Autodesk Inventor part; units mm, degrees
ref_plane "YZ Plane" through (0, 0, 0) normal (1, 0, 0) x (0, 1, 0)
ref_plane "XZ Plane" through (0, 0, 0) normal (0, 1, 0) x (-1, 0, 0)
ref_plane "XY Plane" through (0, 0, 0) normal (0, 0, 1) x (1, 0, 0)
sketch "スケッチ1" plane through (0, 0, 0) normal (0, 1, 0) x (-1, 0, 0)
  line L0 (0, 0) -> (70, 0)
  line L1 (70, 0) -> (70, -170)
  line L2 (70, -170) -> (0, -170)
  line L3 (0, -170) -> (0, 0)
  arc A0 (0, -118.9591) -> (0, -26.9591) centre (0, -72.9591) ccw
  arc A1 (0, -128.9591) -> (0, -16.9591) centre (0, -72.9591) ccw
  line L4 (10, -17.8592) -> (0, -17.8592)
  line L5 (0, -17.8592) -> (0, -2.8592)
  line L6 (0, -2.8592) -> (10, -2.8592)
  line L7 (10, -2.8592) -> (10, -17.8592)
  line L8 (10, -128.0591) -> (0, -128.0591)
  line L9 (0, -128.0591) -> (0, -143.0591)
  line L10 (0, -143.0591) -> (10, -143.0591)
  line L11 (10, -143.0591) -> (10, -128.0591)
  line L12 (54.5871, -60.4591) -> (54.5871, -85.4591)
  point P0 (54.5871, -72.9591)
  point P1 (46, -72.9591)
  dimension "d8" = 70
  dimension "d9" = 170
  dimension "d10" = 46
  dimension "d11" = 56
  dimension "d12" = 10
  dimension "d13" = 10
  dimension "d14" = 15
  dimension "d15" = 15
  dimension "d17" = 25
extrude "押し出し1" add sketch "スケッチ1" along normal blind 81 contours L6 L7 A1 L3 | A1 L4 L3 | L4 A1 L12 L8 L3 A0 | L3 A1 L11 L10 | L3 L8 A1
ref_plane "作業平面1" through (-54.5871, 0, -85.4591) normal (-1, 0, 0) x (0, 0, 1)
sketch "スケッチ2" plane through (-54.5871, 0, -85.4591) normal (-1, 0, 0) x (0, 0, 1)
  line L0 (-33.5, 81) -> (58.5, 81)
  line L1 (0, 60.4) -> (25, 60.4)
  line L2 (25, 60.4) -> (25, 0)
  line L3 (25, 0) -> (0, 0)
  line L4 (0, 0) -> (0, 60.4)
  line L5 (0, 81) -> (25, 81)
  line L6 (0, 0) -> (0, 81)
  line L7 (0, 0) -> (25, 0)
  line L8 (-57.5999, 0) -> (-57.5999, 81)
  line L9 (82.5999, 0) -> (82.5999, 81)
  line L10 (-57.5999, 81) -> (82.5999, 0)
  line L11 (-57.5999, 0) -> (-42.5999, 0)
  line L12 (-57.5999, 0) -> (82.5999, 81)
  line L13 (12.5, 40.5) -> (12.5, 0) construction
  point P0 (85.4591, 0)
  point P1 (12.5, 81)
  point P2 (12.5, 81)
  point P3 (0, 40.5)
  dimension "d21" = 25
  dimension "d22" = 60.4
  dimension "d50" = 20.6
  dimension "d92" = 40.5
  dimension "d93" = 40.5
  dimension "d96" = 12.5
extrude "押し出し2" add sketch "スケッチ2" along normal blind 30 contours L1 L2 L12 L10 L4 | L10 L12 L4 | L2 L10 L12 | L12 L10 L2 L3 L4
ref_plane "作業平面3" through (-84.5871, 0, -85.4591) normal (-1, 0, 0) x (0, 0, 1)
sketch "スケッチ4" plane through (-84.5871, 0, -85.4591) normal (-1, 0, 0) x (0, 0, 1)
  line L0 (2.45, 50.4) -> (22.55, 50.4)
  line L1 (22.55, 50.4) -> (22.55, 10.4)
  line L2 (22.55, 10.4) -> (2.45, 10.4)
  line L3 (2.45, 10.4) -> (2.45, 50.4)
  line L4 (0, 60.4) -> (25, 60.4)
  line L5 (0, 0) -> (0, 60.4)
  line L6 (0, 60.4) -> (0, 0)
  line L7 (0, 0) -> (25, 0)
  line L8 (7.6, 54.5) -> (17.3, 54.5)
  line L9 (7.7, 6.3) -> (17.4, 6.3)
  line L10 (25, 60.4) -> (0, 60.4)
  line L11 (0, 81) -> (25, 81)
  line L12 (25, 0) -> (25, 60.4)
  point P0 (85.4591, 0)
  point P1 (12.5, 50.4)
  point P2 (12.5, 60.4)
  point P3 (2.45, 30.4)
  point P4 (0, 30.2)
  point P5 (0, 0.35)
  point P6 (25, 60)
  point P7 (12.55, 6.3)
  point P8 (12.45, 54.5)
  point P9 (12.5, 60.4)
  point P10 (12.5, 10.4)
  point P11 (12.55, 40.5)
  point P12 (12.5, 81)
  dimension "d28" = 20.1
  dimension "d29" = 40
  dimension "d52" = 10.4
  dimension "d53" = 2.45
  dimension "d54" = 4.1
  dimension "d55" = 4.1
  dimension "d56" = 4.1
  dimension "d57" = 4.1
  dimension "d58" = 9.7
  dimension "d59" = 9.7
  dimension "d100" = 40.5
  dimension "d101" = 9.9
  dimension "d102" = 40.5
  dimension "d107" = 2.45
extrude "押し出し3" cut sketch "スケッチ4" against normal blind 27.5 contours L0 L1 L2 L3
ref_plane "作業平面4" through (-10, 0, -143.0591) normal (-1, 0, 0) x (0, 0, 1)
sketch "スケッチ5" plane through (-10, 0, -143.0591) normal (-1, 0, 0) x (0, 0, 1)
  line L0 (0, 81) -> (15, 81)
  line L1 (0, 0) -> (15, 0)
  line L2 (125.1998, 81) -> (140.1998, 81)
  line L3 (125.1998, 0) -> (140.1998, 0)
  point P0 (143.0591, 0)
  point P1 (7.5, 69)
  point P2 (7.5, 12)
  point P3 (132.6998, 69)
  point P4 (132.6998, 12)
  point P5 (7.5, 81)
  point P6 (7.5, 0)
  point P7 (132.6998, 81)
  point P8 (132.6998, 0)
  dimension "d35" = 0
  dimension "d36" = 0
  dimension "d37" = 0
  dimension "d38" = 0
  dimension "d39" = 12
  dimension "d40" = 12
  dimension "d41" = 12
  dimension "d42" = 12
hole "穴1" at (-10, 69, -135.5591) at (-10, 12, -135.5591) at (-10, 69, -10.3592) at (-10, 12, -10.3592) direction (1, 0, 0) diameter 5 end through all
sketch "スケッチ6" plane through (-84.5871, 0, -85.4591) normal (-1, 0, 0) x (0, 0, 1)
  line L0 (7.7, 6.3) -> (17.4, 6.3)
  line L1 (7.7, 54.5) -> (17.4, 54.5)
  line L2 (22.55, 10.4) -> (2.45, 10.4)
  line L3 (2.45, 50.4) -> (22.55, 50.4)
  point P0 (85.4591, 0)
  point P1 (12.55, 6.3)
  point P2 (12.55, 54.5)
  point P3 (12.5, 10.4)
  point P4 (12.5, 50.4)
  dimension "d63" = 9.7
  dimension "d64" = 9.7
  dimension "d65" = 4.1
  dimension "d66" = 4.1
hole "穴2" at (-84.5871, 54.5, -77.7591) at (-84.5871, 54.5, -68.0591) at (-84.5871, 6.3, -77.7591) at (-84.5871, 6.3, -68.0591) direction (1, 0, 0) diameter 4 depth 10
ref_plane "作業平面5" through (-84.5871, 60.4, -85.4591) normal (0, 1, 0) x (1, 0, 0)
sketch "スケッチ8" plane through (-84.5871, 60.4, -85.4591) normal (0, 1, 0) x (1, 0, 0)
  line L0 (14.2, -17.5) -> (21.2, -17.5)
  line L1 (21.2, -17.5) -> (21.2, -7.5)
  line L2 (21.2, -7.5) -> (14.2, -7.5)
  line L3 (14.2, -7.5) -> (14.2, -17.5)
  line L4 (0, -114.071) -> (0, 86.2117)
  line L5 (30, 0) -> (30, -25)
  point P0 (84.5871, -85.4591)
  point P1 (14.2, -12.5)
  point P2 (30, -12.5)
  dimension "d87" = 7
  dimension "d88" = 10
  dimension "d89" = 14.2
extrude "押し出し5" cut sketch "スケッチ8" against normal blind 12
fillet "フィレット2" radius 1 23 edges at (-10, 40.5, -143.0591) (-10, 81, -135.5591) (-5, 81, -143.0591) (-5, 0, -143.0591) (-10, 0, -135.5591) (-10, 0, -10.3592) (-5, 0, -2.8592) (-69.5871, 0, -85.4591) (-69.5871, 0, -60.4591) (-84.5871, 0, -72.9591) (-84.5871, 30.2, -85.4591) (-69.5871, 60.4, -85.4591) (-84.5871, 60.4, -72.9591) (-84.5871, 30.2, -60.4591) (-69.5871, 60.4, -60.4591) (-38.6854, 0, -32.4692) (-38.6854, 0, -113.4491) (-10, 40.5, -2.8592) (-5, 81, -2.8592) (-10, 81, -10.3592) (-38.6854, 81, -32.4692) (-38.6854, 81, -113.4491) (-54.5871, 81, -72.9591)
sketch "スケッチ9" plane through (-84.5871, 0, -85.4591) normal (-1, 0, 0) x (0, 0, 1)
  line L0 (2.45, 50.4) -> (22.55, 50.4)
  line L1 (2.45, 50.4) -> (22.55, 50.4)
  line L2 (-57.5999, 80) -> (-57.5999, 1)
  line L3 (82.5999, 1) -> (82.5999, 80)
  line L4 (0, 59.4) -> (0, 80)
  line L5 (25, 59.4) -> (25, 80)
  point P0 (85.4591, 0)
  point P1 (12.5, 50.4)
  point P2 (12.5, 50.4)
  point P3 (12.5, 50.4)
  dimension "d103" = 70.0999
  dimension "d104" = 70.0999
  dimension "d105" = 57.5999
  dimension "d106" = 57.5999
properties part number "motor_mount1_3D プリント"
Could you check a few things on this model? Use its own coordinates, in mm. A direction names the side the tool comes from. Coordinates: 2 decimals unless noted, no trailing zeros. Order: outer loops, then holes, each group sorted by start corner. A loop starts at its lowest first (then second) coordinate and runs counter-clockwise, first axis right, second up. Notation, with made-up numbers: (22.5, 38) -> (79.5, 38) arc R11 cw to (79.5, 57) -> close; hole circle Ø8 at (-39.75, 38.5). An arc over 180 degrees is marked (long way). One line per item, written item: value. Start each with the question number.
1) If I drill on L1, parallel to Z at x = -75.5, y = 6; L2, parallel to Z at x = -77.25, y = 54.5; L3, parallel to Z at x = -71, y = 25.5, over which ranges is the centre line in solid material (lowest first)? Write a range as [from, to].
2) Imagine slicing it at A-A on y = 54.5. List the corners of the cut face in (x, z) for me.
3) Which directions (+Z, -Z, +X, -X, +Y, -Y) give clear straight access to the entire face, cutting with the end or side of a thin tool? Please do faces 1 (the flat face through (-10, 40, -135)), 2 (the flat face through (-67, 55, -77.959)), 3 (the flat face through (-47, 81, -68)), 4 (the flat face through (-72, 60.4, -73)), 5 (the cylindrical face through (-79.517, 53.148, -79.233)).
4) I'm going to push flat-ended pins straight in: pin 1 (14.5 mm diameter, centred on x = -73, y = 23, fed in from -Z); pin 2 (5 mm diameter, centred on x = -50, y = 14.5, fed in from -Z); pin 3 (11.5 mm diameter, centred on x = -71, z = -70.5, fed in from +Y); pin 4 (3 mm diameter, centred on y = 12, z = -10.36, fed in from +X). Where does each tip first touch, or does it pass through?
5) Imagine slicing it at B-B on y = 34.5. List the corners of the cut face in (x, z) for me, plus the area to 3 significant figures.
6) Imagine slicing it at C-C on y = 69. List the corners of the cut face in (x, z) for me, plus the area to 3 significant figures.
7) We'd pull the mould along Z, two halves only. Please class faces 6 (the flat face through (-71, 10.4, -73)), 7 (the flat face through (0, 40, -15)), 8 (the flat face through (-69, 30, -85.459)): +Z half, -Z half, draft (parallel to the pull), parting line (faces both ways), or undercut.
8) Imagine slicing it at D-D on y = 6.3. List the corners of the cut face in (x, z) for me, plus the area to 3 significant figures.
Answer list:
1. L1: z = [-85.46, -79.74], [-75.78, -70.04], [-66.08, -60.46]
1. L2: z = [-85.46, -79.76], [-75.76, -70.06], [-66.06, -60.46]
1. L3: z = [-85.46, -83.01], [-62.91, -60.46]
2. outline: (-84.59, -84.46) arc R1 ccw to (-83.59, -85.46) -> (-54.59, -85.46) arc R56 ccw to (-10, -128.06) -> (-10, -142.06) arc R1 ccw to (-9, -143.06) -> (0, -143.06) -> (0, -118.96) arc R46 cw to (0, -26.96) -> (0, -2.86) -> (-9, -2.86) arc R1 ccw to (-10, -3.86) -> (-10, -17.86) arc R56 ccw to (-54.59, -60.46) -> (-83.59, -60.46) arc R1 ccw to (-84.59, -61.46) -> (-84.59, -66.06) -> (-74.59, -66.06) -> (-74.59, -70.06) -> (-84.59, -70.06) -> (-84.59, -75.76) -> (-74.59, -75.76) -> (-74.59, -79.76) -> (-84.59, -79.76) -> close; hole (-70.39, -77.96) -> (-63.39, -77.96) -> (-63.39, -67.96) -> (-70.39, -67.96) -> close
3. face 1: -Z, -X, +Y, -Y
3. face 2: +Y
3. face 3: +Z, -Z, +X, -X, +Y
3. face 4: +Z, -Z, -X, +Y
3. face 5: -X
4. pin 1: stops at z = -85.46
4. pin 2: stops at z = -102.62
4. pin 3: stops at y = 60.4
4. pin 4: passes through
5. outline: (-84.59, -84.46) arc R1 ccw to (-83.59, -85.46) -> (-54.59, -85.46) arc R56 ccw to (-10, -128.06) -> (-10, -142.06) arc R1 ccw to (-9, -143.06) -> (0, -143.06) -> (0, -118.96) arc R46 cw to (0, -26.96) -> (0, -2.86) -> (-9, -2.86) arc R1 ccw to (-10, -3.86) -> (-10, -17.86) arc R56 ccw to (-54.59, -60.46) -> (-83.59, -60.46) arc R1 ccw to (-84.59, -61.46) -> (-84.59, -62.91) -> (-57.09, -62.91) -> (-57.09, -83.01) -> (-84.59, -83.01) -> close
5. area: 2,060 mm2
6. outline: (-54.59, -85.46) arc R56 ccw to (-10, -128.06) -> (-10, -133.06) -> (0, -133.06) -> (0, -118.96) arc R46 cw to (0, -26.96) -> (0, -12.86) -> (-10, -12.86) -> (-10, -17.86) arc R56 ccw to (-54.59, -60.46) -> close; (-10, -142.06) arc R1 ccw to (-9, -143.06) -> (0, -143.06) -> (0, -138.06) -> (-10, -138.06) -> close; (-10, -7.86) -> (0, -7.86) -> (0, -2.86) -> (-9, -2.86) arc R1 ccw to (-10, -3.86) -> close
6. area: 1,770 mm2
7. face 6: undercut
7. face 7: draft
7. face 8: -Z half
8. outline: (-84.59, -84.46) arc R1 ccw to (-83.59, -85.46) -> (-54.59, -85.46) arc R56 ccw to (-10, -128.06) -> (-10, -142.06) arc R1 ccw to (-9, -143.06) -> (0, -143.06) -> (0, -118.96) arc R46 cw to (0, -26.96) -> (0, -2.86) -> (-9, -2.86) arc R1 ccw to (-10, -3.86) -> (-10, -17.86) arc R56 ccw to (-54.59, -60.46) -> (-83.59, -60.46) arc R1 ccw to (-84.59, -61.46) -> (-84.59, -66.06) -> (-74.59, -66.06) -> (-74.59, -70.06) -> (-84.59, -70.06) -> (-84.59, -75.76) -> (-74.59, -75.76) -> (-74.59, -79.76) -> (-84.59, -79.76) -> close
8. area: 2,540 mm2
